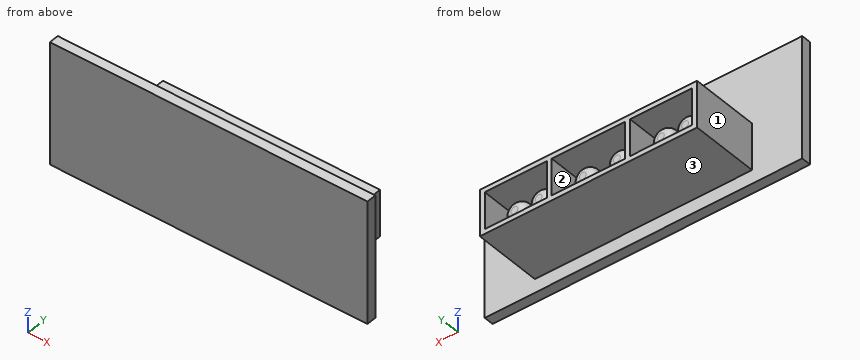
from build123d import *

# Parameters (mm, degrees)
SKETCH1_W           = 65
SKETCH1_H           = 25
BOSS_EXTRUDE1_DEPTH = 2
SKETCH2_W           = 44.45
SKETCH2_H           = 9.525
SKETCH2_W_2         = 12.7
SKETCH2_H_2         = 7.525
SKETCH2_W_3         = 15.049999936
BOSS_EXTRUDE2_DEPTH = 14
SKETCH3_R           = 2.299999953
BOSS_EXTRUDE4_DEPTH = 11.1125
FILLET2_R           = 1.6


with BuildPart() as part:
    # Sketch1 → Boss-Extrude1 (new body)
    with BuildSketch(Plane(origin=(0, 0, 0), x_dir=(1, 0, 0), z_dir=(0, 1, 0))):
        with Locations((-32.5, 12.5)):
            Rectangle(SKETCH1_W, SKETCH1_H)
    extrude(amount=BOSS_EXTRUDE1_DEPTH)

    # Sketch2 → Boss-Extrude2 (add)
    with BuildSketch(Plane(origin=(0, 2, 0), x_dir=(1, 0, 0), z_dir=(0, 1, 0))):
        with Locations((-32.5, 17.4625)):
            Rectangle(SKETCH2_W, SKETCH2_H)
        with Locations((-47.375, 17.4625)):
            Rectangle(SKETCH2_W_2, SKETCH2_H_2, mode=Mode.SUBTRACT)
        with Locations((-17.625, 17.4625)):
            Rectangle(SKETCH2_W_2, SKETCH2_H_2, mode=Mode.SUBTRACT)
        with Locations((-32.5, 17.4625)):
            Rectangle(SKETCH2_W_3, SKETCH2_H_2, mode=Mode.SUBTRACT)
    extrude(amount=BOSS_EXTRUDE2_DEPTH)

    # Sketch3 → Boss-Extrude4 (add)
    with BuildSketch(Plane(origin=(0, 2, 0), x_dir=(1, 0, 0), z_dir=(0, 1, 0))):
        with Locations((-36, 17.4625)):
            Circle(SKETCH3_R)
        with Locations((-49.97, 17.4625)):
            Circle(SKETCH3_R)
        with Locations((-19.998, 17.4625)):
            Circle(SKETCH3_R)
        with Locations((-29, 17.4625)):
            Circle(SKETCH3_R)
        with Locations((-15.03, 17.4625)):
            Circle(SKETCH3_R)
        with Locations((-45.002, 17.4625)):
            Circle(SKETCH3_R)
    extrude(amount=BOSS_EXTRUDE4_DEPTH)

    # Fillet2
    fillet2_edges = [part.edges().sort_by_distance(p)[0] for p in [
        (-38.299999953, 13.1125, -17.4625),
        (-52.269999953, 13.1125, -17.4625),
        (-22.297999953, 13.1125, -17.4625),
        (-31.299999953, 13.1125, -17.4625),
        (-17.329999953, 13.1125, -17.4625),
        (-47.301999953, 13.1125, -17.4625),
    ]]
    fillet(fillet2_edges, radius=FILLET2_R)


solid = part.part
Verification items for the finished model (mm, model axes). Face numbers are marked on the shaded views. A direction names the side the tool comes from. Coordinates: 2 decimals unless noted, no trailing zeros. Order: outer loops, then holes, each group sorted by start corner. A loop starts at its lowest first (then second) coordinate and runs counter-clockwise, first axis right, second up.
1. Sectioned sample at B-B, the plane y = 8.25. Give the number of separate pieces and of enclosed holes in the cut face, and give its area (3 significant figures).
Results found:
separate pieces: 7
enclosed holes: 3
area: 219 mm2
2. Scan lines: line 1 (Z direction, x = -45, y = 2.25) (1 decimal); line 2 (X direction, y = 10.25, z = -14.75) (3 decimals); line 3 (Z direction, x = -12.5, y = 3.75) (3 decimals). Record each from-to range of solid material in increasing order.
Results found:
line 1: z = -22.2 to -21.2, -19.8 to -15.2, -13.7 to -12.7
line 2: x = -54.725 to -53.725, -41.025 to -40.025, -24.975 to -23.975, -11.275 to -10.275
line 3: z = -22.225 to -21.225, -13.7 to -12.7
3. Sectioned sample at C-C, the plane z = -10.5. Record the cut outline in (x, y).
Results found:
outline: (-65, 0) - (0, 0) - (0, 2) - (-65, 2) - close
4. Sectioned sample at D-D, the plane x = -59.5. Record the cut outline in (y, z).
Results found:
outline: (0, -25) - (2, -25) - (2, 0) - (0, 0) - close
5. Sectioned sample at A-A, the plane y = 14.5. Record the cut outline in (x, z) (3 decimals).
Results found:
outline: (-54.725, -22.225) - (-10.275, -22.225) - (-10.275, -12.7) - (-54.725, -12.7) - close; hole (-53.725, -21.225) - (-41.025, -21.225) - (-41.025, -13.7) - (-53.725, -13.7) - close; hole (-40.025, -21.225) - (-24.975, -21.225) - (-24.975, -13.7) - (-40.025, -13.7) - close; hole (-23.975, -21.225) - (-11.275, -21.225) - (-11.275, -13.7) - (-23.975, -13.7) - close
6. Go/stop test with flat-tipped pins: pin 1 Ø3 at (y, z) = (10.5, -21.5) entering from +X (3 decimals); pin 2 Ø2 at (x, z) = (-7, -12.5) entering from +Y; pin 3 Ø6 at (y, z) = (9, -17.5) entering from -X (3 decimals). Record where each tip stops, or that it passes through.
Results found:
pin 1: stops at x = -10.275
pin 2: stops at y = 2
pin 3: stops at x = -54.725
7. Set-up check for the marked faces 1, 2 and 3: record each of +Z, -Z, +X, -X, +Y, -Y from which the full face is reachable in a straight line by a thin tool's end or side.
Results found:
face 1: +Z, -Z, -X, +Y
face 2: +Y
face 3: -Z, +X, -X, +Y
